from build123d import *

# Parameters (mm, degrees)
BOSS_EXTRUDE6_DEPTH = 37.5
BOSS_EXTRUDE1_DEPTH = 10.16
CUT_EXTRUDE4_DEPTH  = 14


with BuildPart() as part:
    # Sketch15 → Boss-Extrude6 (new, symmetric)
    with BuildSketch(Plane(origin=(0, 0, 0), x_dir=(1, 0, 0), z_dir=(0, 1, 0))):
        with BuildLine():
            Line((-5.617617549, 4.264), (-9.385342517, 4.264))
            ThreePointArc((-9.385342517, 4.264), (-9.881519345, 4.469523172), (-10.087042517, 4.9657))
            Line((-10.087042517, 4.9657), (-10.087042517, 5.533957914))
            ThreePointArc((-10.087042517, 5.533957914), (-10.03362862, 5.802487278), (-9.881518735, 6.030135353))
            Line((-9.881518735, 6.030135353), (-5.15064406, 10.76099839))
            ThreePointArc((-5.15064406, 10.76099839), (-3.674584079, 11.747268168), (-1.933453584, 12.0936))
            Line((-1.933453584, 12.0936), (1.933453584, 12.0936))
            ThreePointArc((1.933453584, 12.0936), (3.674584079, 11.747268168), (5.15064406, 10.76099839))
            Line((5.15064406, 10.76099839), (9.881518735, 6.030135353))
            ThreePointArc((9.881518735, 6.030135353), (10.03362862, 5.802487278), (10.087042517, 5.533957914))
            Line((10.087042517, 5.533957914), (10.087042517, 4.9657))
            ThreePointArc((10.087042517, 4.9657), (9.881519345, 4.469523172), (9.385342517, 4.264))
            Line((9.385342517, 4.264), (5.617617549, 4.264))
            Line((5.617617549, 4.264), (-5.617617549, 4.264))
        make_face()
    extrude(amount=BOSS_EXTRUDE6_DEPTH, both=True)

    # Sketch1 → Boss-Extrude1 (add, symmetric)
    with BuildSketch(Plane(origin=(0, 0, 0), x_dir=(1, 0, 0), z_dir=(0, 1, 0))):
        with BuildLine():
            Line((-14.587702875, -0.2), (-14.587702875, -20))
            Line((-14.587702875, -20), (7, -20))
            Line((7, -20), (7, -0.2))
            Line((7, -0.2), (5.617617549, -0.2))
            ThreePointArc((5.617617549, -0.2), (4.377622689, 0.313622689), (3.864, 1.553617549))
            Line((3.864, 1.553617549), (3.864, 2.510382451))
            ThreePointArc((3.864, 2.510382451), (4.377622689, 3.750377311), (5.617617549, 4.264))
            Line((5.617617549, 4.264), (5.617617549, 5))
            Line((5.617617549, 5), (-5.617617549, 5))
            Line((-5.617617549, 5), (-5.617617549, 4.264))
            ThreePointArc((-5.617617549, 4.264), (-4.377622689, 3.750377311), (-3.864, 2.510382451))
            Line((-3.864, 2.510382451), (-3.864, 1.553617549))
            ThreePointArc((-3.864, 1.553617549), (-4.377622689, 0.313622689), (-5.617617549, -0.2))
            Line((-5.617617549, -0.2), (-8.236278456, -0.2))
            ThreePointArc((-8.236278456, -0.2), (-8.736202395, 0.29992394), (-9.236126335, -0.2))
            Line((-9.236126335, -0.2), (-14.587702875, -0.2))
        make_face()
    extrude(amount=BOSS_EXTRUDE1_DEPTH, both=True)

    # Sketch12 → Cut-Extrude4 (cut)
    with BuildSketch(Plane(origin=(7, 0, 0), x_dir=(0, 0, -1), z_dir=(1, 0, 0))):
        Polygon((-22.36, 7.874), (-22.36, -7.874), (-13.36, -7.874), (-13.36, -6.604), (-8.534, -6.604), (-8.534, -7.874), (-3.2, -7.874), (-3.2, 7.874), (-8.534, 7.874), (-8.534, 6.604), (-13.36, 6.604), (-13.36, 7.874), align=None)
    extrude(amount=-CUT_EXTRUDE4_DEPTH, mode=Mode.SUBTRACT)


solid = part.part
Design review of the part built by this model. Coordinates are the model's own, in mm. A direction names the side the tool comes from. Round coordinates to 2 decimals unless told otherwise and drop trailing zeros. Write each loop counter-clockwise with the first axis right and the second up, starting at its lowest first coordinate (ties: lowest second). Pieces come first, ordered by that corner, then holes. Notation, with made-up numbers: (50.25, 80) -> (104.25, 80) arc R8 cw to (104.25, 90) -> close; hole circle Ø6 at (-36, -23). An arc over 180 degrees is marked (long way). One line per item, written item: value. Start each with the question number.
Q1. Tool access review of faces 1 (the face through (7, 1, 3)), 2 (the face through (0, -7.874, 17)), 3 (the face through (-4, 10.16, 8)), 4 (the face through (-4.36, 0.14, -0.33)): name each direction out of +Z, -Z, +X, -X, +Y, -Y from which nothing blocks a thin tool from reaching the whole face with its end or side.
Q2. Add section A-A (y = -2.5). Give the boundary of the cut face in (x, z).
Q3. Add section C-C (x = -11.5). Give the boundary of the cut face in (y, z), then the cut area to 3 significant figures.
Q4. Add section D-D (y = 22). Give the boundary of the cut face in (x, z).
Q5. Insertion check: P1, Ø5, axis at x = 5, z = 5.5, coming from the -Y side; P2, Ø3, axis at x = -7, y = 3, coming from the -Z side; P3, Ø1, axis at x = -2, y = -7, coming from the +Z side. Each pin has a flat end and moves straight along its axis. Give the tip position at first contact, or say it passes through.
Q6. The part is to be moulded in two halves that separate along Y. For faces 5 (the face through (0, -6.604, 11)), 6 (the face through (0, 37.5, -7)), 7 (the face through (-7, 0, 12)), 8 (the face through (4.364, 0.142, -3.737)), say which applies: pulls with the +Y half, pulls with the -Y half, needs draft (parallel to the pull), parting line crosses it, or undercut.
Q7. Add section B-B (z = 6.5). Give the boundary of the cut face in (x, y).
Q8. To check wall thickness, follow probe 1 along Y at (x, z) = (-2, 14); probe 2 along X at (y, z) = (6, 14); probe 3 along X at (y, z) = (10, 2). State the ranges of each line that lie inside material, in increasing order.
Response:
1. face 1: +Z, +X, +Y, -Y
1. face 2: +Z, +X
1. face 3: +Z, +X, -X, +Y
1. face 4: +Y, -Y
2. outline: (-14.59, 0.2) -> (-9.24, 0.2) arc R0.5 ccw to (-8.24, 0.2) -> (-5.62, 0.2) arc R1.75 cw to (-3.86, -1.55) -> (-3.86, -2.51) arc R1.75 cw to (-5.62, -4.26) -> (-9.39, -4.26) arc R0.7 ccw to (-10.09, -4.97) -> (-10.09, -5.53) arc R0.7 ccw to (-9.88, -6.03) -> (-5.15, -10.76) arc R4.55 ccw to (-1.93, -12.09) -> (1.93, -12.09) arc R4.55 ccw to (5.15, -10.76) -> (9.88, -6.03) arc R0.7 ccw to (10.09, -5.53) -> (10.09, -4.97) arc R0.7 ccw to (9.39, -4.26) -> (5.62, -4.26) arc R1.75 cw to (3.86, -2.51) -> (3.86, -1.55) arc R1.75 cw to (5.62, 0.2) -> (7, 0.2) -> (7, 3.2) -> (-7, 3.2) -> (-7, 20) -> (-14.59, 20) -> close
3. outline: (-10.16, 0.2) -> (10.16, 0.2) -> (10.16, 20) -> (-10.16, 20) -> close
3. area: 402 mm^2
4. outline: (-10.09, -5.53) arc R0.7 ccw to (-9.88, -6.03) -> (-5.15, -10.76) arc R4.55 ccw to (-1.93, -12.09) -> (1.93, -12.09) arc R4.55 ccw to (5.15, -10.76) -> (9.88, -6.03) arc R0.7 ccw to (10.09, -5.53) -> (10.09, -4.97) arc R0.7 ccw to (9.39, -4.26) -> (-9.39, -4.26) arc R0.7 ccw to (-10.09, -4.97) -> close
5. P1: stops at y = -10.16
5. P2: stops at z = -10.41
5. P3: stops at z = 13.36
6. face 5: undercut
6. face 6: pulls with the +Y half
6. face 7: undercut
6. face 8: needs draft
7. outline: (-14.59, -10.16) -> (7, -10.16) -> (7, -7.87) -> (-7, -7.87) -> (-7, 7.87) -> (7, 7.87) -> (7, 10.16) -> (-14.59, 10.16) -> close
8. probe 1: y = -10.16 to -7.87, 7.87 to 10.16
8. probe 2: x = -14.59 to -7
8. probe 3: x = -14.59 to 7
